Print and shaded views of the part. All mm, measured from the part's lowest x, y and z. Coordinates: 2 decimals unless noted, no trailing zeros. Write each loop counter-clockwise with the first axis right and the second up, starting at its lowest first coordinate (ties: lowest second). Pieces come first, ordered by that corner, then holes. Notation, with made-up numbers: (27.25, -34) -> (84.25, -34) arc R20 ccw to (84.25, -27) -> close; hole circle Ø9 at (32, 16.5). An arc over 180 degrees is marked (long way). Write item = value, one per line.
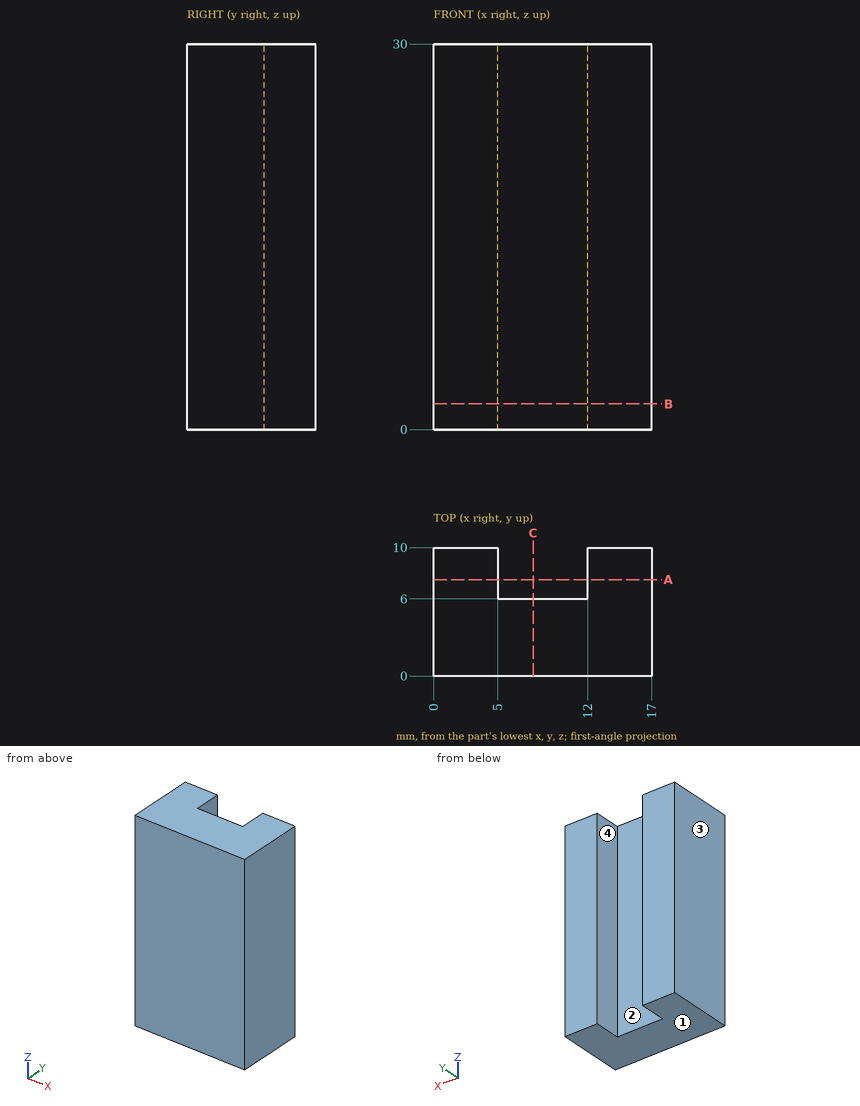
Q1. Saw through at B-B on z = 2. Give the cut face in (x, y).
Model answer:
outline = (0, 0) -> (17, 0) -> (17, 10) -> (12, 10) -> (12, 6) -> (5, 6) -> (5, 10) -> (0, 10) -> close
Q2. Pin check, flat tip, straight feed: pin 1 (3.5 mm diameter, centred on x = 7.5, z = 19.5, fed in from +Y). Stop position of the tip, or through.
Model answer:
pin_1 = 6
Q3. Saw through at C-C on x = 7.75. Give the cut face in (y, z), and give its area (3 significant figures).
Model answer:
outline = (0, 0) -> (6, 0) -> (6, 30) -> (0, 30) -> close
area = 180 mm²
Q4. Probe line 1 (X direction, y = 9, z = 9.5); line 2 (Y direction, x = 9, z = 14.5). List the from-to ranges inside material, lowest first. Write a range as from..to.
Model answer:
line_1 = 0..5, 12..17
line_2 = 0..6
Q5. Mould opens along X. For the marked faces 1, 2, 3 and 4 say: released by +X, released by -X, zero draft, split by the parting line, or undercut.
Model answer:
face_1 = zero draft
face_2 = undercut
face_3 = released by -X
face_4 = undercut
Q6. Saw through at A-A on y = 7.5. Give the cut face in (x, z), and give its area (3 significant figures).
Model answer:
outline = (0, 0) -> (5, 0) -> (5, 30) -> (0, 30) -> close; (12, 0) -> (17, 0) -> (17, 30) -> (12, 30) -> close
area = 300 mm²
